Verification items for the finished model (mm, model axes). A direction names the side the tool comes from. Round coordinates to 2 decimals unless told otherwise and drop trailing zeros. Order: outer loops, then holes, each group sorted by start corner. A loop starts at its lowest first (then second) coordinate and runs counter-clockwise, first axis right, second up. Notation, with made-up numbers: M 74.25,26.5 L 78.25,26.5 A33 cw 78.25,60.5 Z; hole C 18.5,43 d10. An arc over 180 degrees is marked long. Write item = value, one per line. Start each with the question number.
from build123d import *

# Parameters (mm, degrees)
SKETCH1_W                      = 8.75
SKETCH1_H                      = 15
BASE_FLANGE1_DEPTH             = 1.75
EDGE_FLANGE1_STRIP_W           = 9.3368
EDGE_FLANGE1_STRIP_H           = 1.75
EDGE_FLANGE1_STRIP_CUT_DEPTH   = 15
EDGE_FLANGE1_DEPTH             = 15
M3_CLEARANCE_HOLE1_D           = 3.4
M3_CLEARANCE_HOLE1_ON_FACE_2_D = 3.4


# Sheet-metal steps are written as plain solids
with BuildPart() as part:
    # Sketch1 → Base-Flange1 (new body)
    with BuildSketch(Plane.XY):
        with Locations((4.375, 7.5)):
            Rectangle(SKETCH1_W, SKETCH1_H)
    extrude(amount=-BASE_FLANGE1_DEPTH)

    # Edge-Flange1 strip (across the edge) → Edge-Flange1 strip cut (cut)
    with BuildSketch(Plane.XZ.offset(-15)):
        with Locations((-3.5, -0.875)):
            Rectangle(EDGE_FLANGE1_STRIP_W, EDGE_FLANGE1_STRIP_H)
    extrude(amount=EDGE_FLANGE1_STRIP_CUT_DEPTH, mode=Mode.SUBTRACT)

    # Edge-Flange1 section (across the edge) → Edge-Flange1 (add)
    with BuildSketch(Plane.XZ.offset(-15)):
        with BuildLine():
            Line((-1.75, 1.1684), (-1.75, 8.75))
            Line((-1.75, 8.75), (0, 8.75))
            Line((0, 8.75), (0, 1.1684))
            ThreePointArc((0, 1.1684), (0.342216437, 0.342216437), (1.1684, 0))
            Line((1.1684, 0), (1.1684, -1.75))
            ThreePointArc((1.1684, -1.75), (-0.89522043, -0.89522043), (-1.75, 1.1684))
        make_face()
    extrude(amount=EDGE_FLANGE1_DEPTH)

    # M3 Clearance Hole1 (through all)
    with Locations(Plane(origin=(-1.75, 10.625, 4.9592), x_dir=(0, 0, -1), z_dir=(-1, 0, 0))):
        with Locations((0, 0), (0, 6.25)):
            Hole(M3_CLEARANCE_HOLE1_D / 2)

    # M3 Clearance Hole1 on face 2 (through all)
    with Locations(Plane(origin=(4.9592, 10.625, -1.75), x_dir=(-1, 0, 0), z_dir=(0, 0, -1))):
        with Locations((0, 0), (0, -6.25)):
            Hole(M3_CLEARANCE_HOLE1_ON_FACE_2_D / 2)


solid = part.part
1) Cross-section at D-D, the plane y = 4. Enter the section's corners in (x, z), then the cut area to 3 significant figures.
2) Gauge pin test, flat ends, axial feed: P1, Ø1, axis at y = 2, z = 7.5, coming from the +X side; P2, Ø3, axis at x = 4.96, y = 10.62, coming from the -Z side; P3, Ø2, axis at x = 4, y = 8.5, coming from the +Z side. Record the tip position at first contact, or that the pin passes through.
3) Cross-section at C-C, the plane x = 6.25. Enter the section's corners in (y, z), then the cut area to 3 significant figures.
4) Release check for a two-part mould opening along Z. For faces 3 (the cylindrical face through (0.333, 7.605, 0.351)), 4 (the cylindrical face through (6.53, 3.72, -0.86)), 5 (the cylindrical face through (-0.86, 11.28, 6.53)) record: pulls with the +Z half, pulls with the -Z half, needs draft (parallel to the pull), parting line crosses it, or undercut.
5) Scan lines: probe 1 along X at (y, z) = (6.75, 6.75); probe 2 along X at (y, z) = (5.25, -0.75). Record each from-to range of solid material in increasing order.
6) Cross-section at A-A, the plane z = 4.25. Enter the section's corners in (x, y), then the cut area to 3 significant figures.
7) Access from +Z, -Z, +X, -X, +Y, -Y to the whole of each face (thin tool, end or side, straight path). Record for faces 1 (the cylindrical face through (-0.87, 7.6, -0.92)), 2 (the flat face through (0, 8, 5)).
8) Cross-section at B-B, the plane y = 1.5. Enter the section's corners in (x, z), then the cut area to 3 significant figures.
Geometry results:
q1.outline = M -1.75,1.17 A2.92 ccw 1.17,-1.75 L 3.3,-1.75 L 3.3,0 L 1.17,0 A1.17 cw 0,1.17 L 0,3.3 L -1.75,3.3 Z; M -1.75,6.62 L 0,6.62 L 0,8.75 L -1.75,8.75 Z; M 6.62,-1.75 L 8.75,-1.75 L 8.75,0 L 6.62,0 Z
q1.area = 20.5 mm^2
q2.P1 = 0
q2.P2 = through
q2.P3 = 0
q3.outline = M 0,-1.75 L 3.27,-1.75 L 3.27,0 L 0,0 Z; M 5.48,-1.75 L 9.52,-1.75 L 9.52,0 L 5.48,0 Z; M 11.73,-1.75 L 15,-1.75 L 15,0 L 11.73,0 Z
q3.area = 18.5 mm^2
q4.face_3 = pulls with the +Z half
q4.face_4 = needs draft
q4.face_5 = undercut
q5.probe_1 = -1.75 to 0
q5.probe_2 = -1.03 to 3.5, 6.42 to 8.75
q6.outline = M -1.75,0 L 0,0 L 0,2.83 L -1.75,2.83 Z; M -1.75,5.92 L 0,5.92 L 0,9.08 L -1.75,9.08 Z; M -1.75,12.17 L 0,12.17 L 0,15 L -1.75,15 Z
q6.area = 15.4 mm^2
q7.face_1 = -Z, -X, +Y, -Y
q7.face_2 = +Z, +X, +Y, -Y
q8.outline = M -1.75,1.17 A2.92 ccw 1.17,-1.75 L 8.75,-1.75 L 8.75,0 L 1.17,0 A1.17 cw 0,1.17 L 0,8.75 L -1.75,8.75 Z
q8.area = 32.2 mm^2
